Read the model definition and answer for the solid it produces. Units are mm, in the model's axes. A direction names the side the tool comes from. Give positions to 0.01 mm unless a question says otherwise; leave off trailing zeros. Write each loop counter-clockwise with the first axis right and the second up, starting at its lowest first coordinate (ties: lowest second). Pieces come first, ordered by that corner, then holes. Notation, with made-up numbers: (-16.5, 18) - (40.5, 18) arc R19 ccw to (40.5, 22) - close; hole circle Ø3 at (28.5, 38). An arc over 180 degrees is marked (long way). Use CSV: the item, a comma, the result in double quotes. Start each with the question number.
from build123d import *

# Parameters (mm, degrees)
BOSS_EXTRUDE1_DEPTH = 38
BOSS_EXTRUDE2_DEPTH = 38


with BuildPart() as part:
    # Sketch1 → Revolve1 (revolve)
    with BuildSketch(Plane.XY):
        Polygon((-41.446882046, 0), (-41.446882046, 35), (3.553117954, 35), (3.553117954, 18.2), (363.553117954, 18.2), (363.553117954, 35), (408.553117954, 35), (408.553117954, 0), align=None)
    revolve(axis=Axis((408.553117954, 0, 0), (-1, 0, 0)))

    # Sketch2 → Boss-Extrude1 (add)
    with BuildSketch(Plane.XY):
        with BuildLine():
            Line((34.62755495, 6.710806587), (42.139274487, 15.00946817))
            ThreePointArc((42.139274487, 15.00946817), (49.553117954, 18.298661583), (56.966961421, 15.00946817))
            Line((56.966961421, 15.00946817), (64.478680957, 6.710806587))
            ThreePointArc((64.478680957, 6.710806587), (67.06483749, 0), (64.478680957, -6.710806587))
            Line((64.478680957, -6.710806587), (56.966961421, -15.00946817))
            ThreePointArc((56.966961421, -15.00946817), (49.553117954, -18.298661583), (42.139274487, -15.00946817))
            Line((42.139274487, -15.00946817), (34.62755495, -6.710806587))
            ThreePointArc((34.62755495, -6.710806587), (32.041398417, 0), (34.62755495, 6.710806587))
        make_face()
    extrude(amount=BOSS_EXTRUDE1_DEPTH)

    # Sketch4 → Boss-Extrude2 (add)
    with BuildSketch(Plane(origin=(0, 0, 0), x_dir=(1, 0, 0), z_dir=(0, 1, 0))):
        with BuildLine():
            Line((20.785581303, 7.29733528), (28.297300839, 15.595996863))
            ThreePointArc((28.297300839, 15.595996863), (35.711144306, 18.885190277), (43.124987774, 15.595996863))
            Line((43.124987774, 15.595996863), (50.63670731, 7.29733528))
            ThreePointArc((50.63670731, 7.29733528), (53.222863843, 0.586528694), (50.63670731, -6.124277893))
            Line((50.63670731, -6.124277893), (43.124987774, -14.422939476))
            ThreePointArc((43.124987774, -14.422939476), (35.711144306, -17.712132889), (28.297300839, -14.422939476))
            Line((28.297300839, -14.422939476), (20.785581303, -6.124277893))
            ThreePointArc((20.785581303, -6.124277893), (18.19942477, 0.586528694), (20.785581303, 7.29733528))
        make_face()
    extrude(amount=BOSS_EXTRUDE2_DEPTH)


solid = part.part
(1) The part is cut by section D-D on x = -14. Write down the section's boundary in (y, z), plus the area to 3 significant figures.
(2) The part is cut by section B-B on y = -22.5. Write down the section's boundary in (x, z), plus the area to 3 significant figures.
(3) Consider probe 1 along X at (y, z) = (-10.5, 19.5); probe 2 along X at (y, z) = (0, -27); probe 3 along X at (y, z) = (32, 11). Determine where each line is inside the solid, lowest interval first.
(4) Given P1, Ø8, axis at x = 190, z = 15.5, coming from the -Y side; P2, Ø8, axis at x = 17, z = -20.5, coming from the -Y side; P3, Ø8, axis at x = 324.5, y = -7, coming from the +Z side; P4, Ø12, axis at x = 190, y = -25, coming from the +Z side, each flat-ended and moving along its own axis, determine where each tip first touches the part or whether it passes through.
(5) For a pull along X with two mould halves and no side action, classify faces 1 (the face through (50, 0, 38)), 2 (the face through (38.44, -10.92, 27.03)), 3 (the face through (408.553, 0, 0)) as pulls with the +X half, pulls with the -X half, needs draft (parallel to the pull), parting line crosses it, or undercut.
(6) Which of the six approach directions +Z, -Z, +X, -X, +Y, -Y give full straight-line access (tool end or side, diameter ignored) to faces 4 (the face through (60.67, 10.92, 27.03)), 5 (the face through (60.775, -10.802, 27.031)), 6 (the face through (186.073, -13.414, -12.3)), 7 (the face through (46.83, 26.67, -11.5)), 8 (the face through (67.064, 0.103, 27.311))?
(7) The part is cut by section A-A on z = 25.5. Write down the section's boundary in (x, y).
(8) The part is cut by section C-C on x = 235.5. Write down the section's boundary in (y, z), plus the area to 3 significant figures.
Reported:
1,outline,"circle Ø70 at (0, 0)"
1,area,"3,850 mm²"
2,outline,"(-41.45, -26.81) - (3.55, -26.81) - (3.55, 26.81) - (-41.45, 26.81) - close; (363.55, -26.81) - (408.55, -26.81) - (408.55, 26.81) - (363.55, 26.81) - close"
2,area,"4,830 mm²"
3,probe 1,"-41.45 to 3.55, 38.06 to 61.05, 363.55 to 408.55"
3,probe 2,"-41.45 to 3.55, 363.55 to 408.55"
3,probe 3,"-41.45 to 3.55, 25.2 to 46.22, 363.55 to 408.55"
4,P1,"y = -14.11"
4,P2,"y = -7.68"
4,P3,"z = 17.95"
4,P4,"through"
5,face 1,"needs draft"
5,face 2,"undercut"
5,face 3,"pulls with the +X half"
6,face 4,"+Z, +Y"
6,face 5,"+Z, -Y"
6,face 6,"none"
6,face 7,"-Z, +Y"
6,face 8,"+Z"
7,outline,"(-41.45, -23.97) - (3.55, -23.97) - (3.55, 23.97) - (-41.45, 23.97) - close; (34.63, -6.71) - (42.14, -15.01) arc R10 ccw to (56.97, -15.01) - (64.48, -6.71) arc R10 ccw to (64.48, 6.71) - (56.97, 15.01) arc R10 ccw to (42.14, 15.01) - (34.63, 6.71) arc R10 ccw to start; (363.55, -23.97) - (408.55, -23.97) - (408.55, 23.97) - (363.55, 23.97) - close"
8,outline,"circle Ø36.4 at (0, 0)"
8,area,"1,040 mm²"
